Model file for the job. Use its own axes, mm. Face numbers are marked on the shaded views. Round coordinates to 2 decimals unless told otherwise and drop trailing zeros. Loops run counter-clockwise (first coordinate to the right, second up) from the corner with the lowest first, then second, coordinate; pieces in that order, holes last. Notation, with made-up numbers: M 40,45.5 L 79,45.5 A10 cw 79,60.5 Z; hole C 43,52.5 d2. An arc over 180 degrees is marked long. Answer in a Markdown table with one row per item.
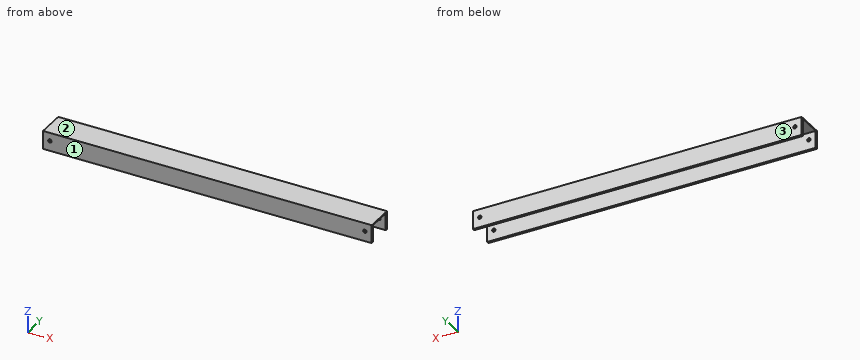
from build123d import *

# Parameters (mm, degrees)
F0_W     = 914.4
F0_H     = 50.8
F1_DEPTH = 6.35
F2_W     = 914.4
F2_H     = 69.85
F3_DEPTH = 3.175
F4_W     = 914.4
F4_H     = 6.35
F5_DEPTH = 47.625
F7_D     = 9.525


with BuildPart() as f1:
    # F0 (on Front) → F1 (new body)
    with BuildSketch(Plane.XZ):
        with Locations((564.6889274399, 584.2)):
            Rectangle(F0_W, F0_H)
    extrude(amount=F1_DEPTH)

    # F2 (on face) → F3 (join)
    with BuildSketch(Plane.XY.offset(609.6)):
        with Locations((564.6889274399, 34.925)):
            Rectangle(F2_W, F2_H)
    extrude(amount=-F3_DEPTH)

    # F4 (on face) → F5 (join, through all)
    with BuildSketch(Plane(origin=(0, 0, 606.425), x_dir=(1, 0, 0), z_dir=(0, 0, -1))):
        with Locations((564.6889274399, -66.675)):
            Rectangle(F4_W, F4_H)
    extrude(amount=F5_DEPTH)

    # F7 (through all)
    with Locations(Plane.XZ.offset(6.35)):
        with Locations((126.5389274399, 586.8924), (1002.8389274399, 586.8924)):
            Hole(F7_D / 2)


solid = f1.part
1. Mould opens along Y. For the marked faces 1, 2 and 3 say: +Y half, -Y half, draft (parallel to the pull), parting line (faces both ways), or undercut.
Verdict:
| item | result |
|---|---|
| face 1 | -Y half |
| face 2 | draft |
| face 3 | +Y half |
2. Saw through at B-B (y = 40.5). Write the cut outline in (x, z) (3 decimals), and give its area (3 significant figures).
Verdict:
| item | result |
|---|---|
| outline | M 107.489,606.425 L 1021.889,606.425 L 1021.889,609.6 L 107.489,609.6 Z |
| area | 2,900 mm² |
3. Wall check: probe 1 along Y at (x, z) = (545, 582); probe 2 along Z at (x, y) = (894, 25) (3 decimals). Give the ranges that are in metal, low to high.
Verdict:
| item | result |
|---|---|
| probe 1 | y = -6.35 to 0, 63.5 to 69.85 |
| probe 2 | z = 606.425 to 609.6 |
4. Saw through at A-A (x = 354). Write the cut outline in (y, z) (3 decimals).
Verdict:
| item | result |
|---|---|
| outline | M -6.35,558.8 L 0,558.8 L 0,606.425 L 63.5,606.425 L 63.5,558.8 L 69.85,558.8 L 69.85,609.6 L -6.35,609.6 Z |
5. Pin check, flat tips, straight feed: pin 1 (7.5 mm diameter, centred on x = 126.54, z = 586.89, fed in from -Y); pin 2 (8 mm diameter, centred on x = 666, y = 44.5, fed in from -Z) (3 decimals). Stop position of each tip, or through.
Verdict:
| item | result |
|---|---|
| pin 1 | passes through |
| pin 2 | stops at z = 606.425 |
